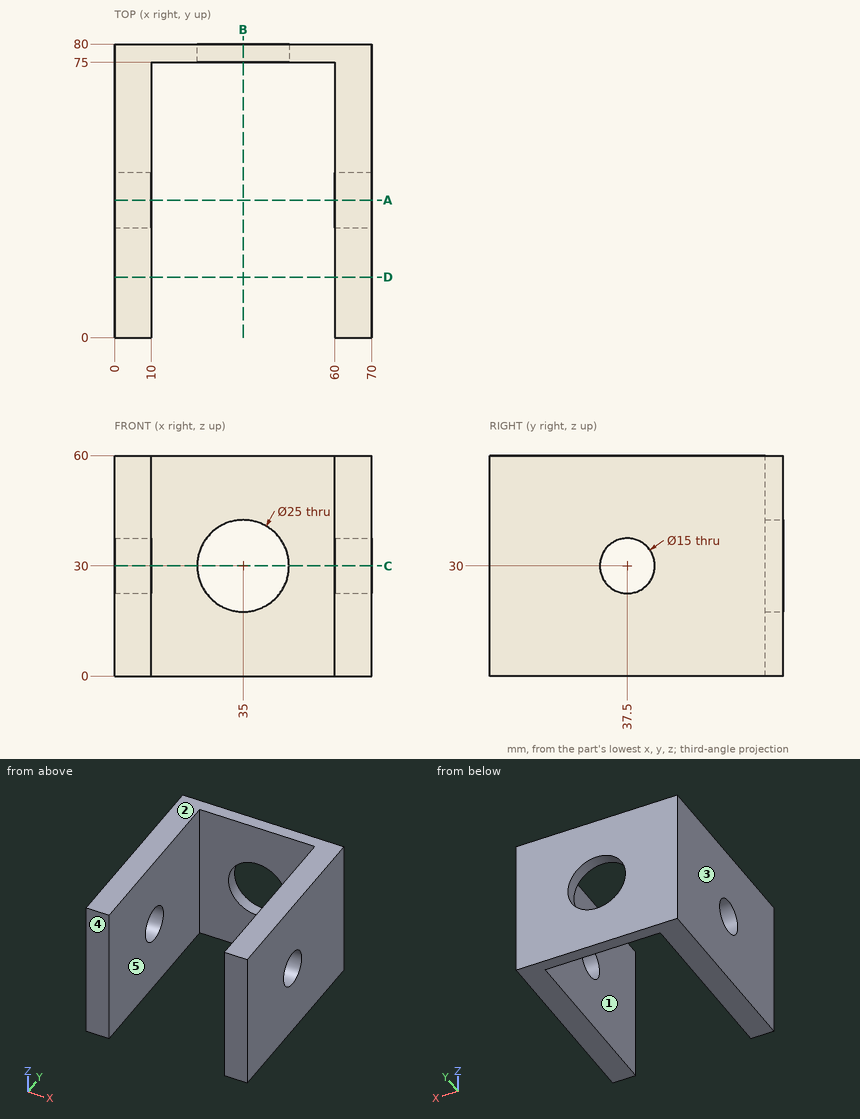
Source: three-view drawing plus pictorial views. Frame: mm from the lowest corner of the part. A direction names the side the tool comes from. Give positions to 0.01 mm unless a question says otherwise; leave off trailing zeros. Order: outer loops, then holes, each group sorted by start corner. A loop starts at its lowest first (then second) coordinate and runs counter-clockwise, first axis right, second up.
1. Mould query, pull axis X, two halves, no side actions, for the marked faces 3, 4 and 5. Classes: released by +X, released by -X, zero draft, split by the parting line, or undercut.
Derived:
face 3: released by -X
face 4: zero draft
face 5: undercut
2. Section D-D on y = 16.5. Return the cut outline in (x, z), and give its area (3 significant figures).
Derived:
outline: (0, 0) - (10, 0) - (10, 60) - (0, 60) - close; (60, 0) - (70, 0) - (70, 60) - (60, 60) - close
area: 1,200 mm2
3. Material intervals for L1, parallel to X at y = 22.5, z = 32; L2, parallel to Z at x = 35, y = 76.2; L3, parallel to Z at x = 64.75, y = 37.5, sorted ascending.
Derived:
L1: x = 0 to 10, 60 to 70
L2: z = 0 to 17.5, 42.5 to 60
L3: z = 0 to 22.5, 37.5 to 60
4. Pin query (flat end, axial travel): pin 1 (1 mm diameter, centred on x = 62, y = 71, fed in from -Z). Return the tip coordinate at first contact, or that it passes through.
Derived:
pin 1: stops at z = 0
5. Reachability of the marked faces 1 and 2 from +Z, -Z, +X, -X, +Y, -Y: full face, straight path, thin tool, end or side. Return the list, or none.
Derived:
face 1: +Z, -Z, -Y
face 2: +Z, +X, -X, +Y, -Y
6. Section C-C on z = 30. Return the cut outline in (x, y).
Derived:
outline: (0, 0) - (10, 0) - (10, 30) - (0, 30) - close; (0, 45) - (10, 45) - (10, 75) - (22.5, 75) - (22.5, 80) - (0, 80) - close; (47.5, 75) - (60, 75) - (60, 45) - (70, 45) - (70, 80) - (47.5, 80) - close; (60, 0) - (70, 0) - (70, 30) - (60, 30) - close
7. Section B-B on x = 35. Return the cut outline in (y, z).
Derived:
outline: (75, 0) - (80, 0) - (80, 17.5) - (75, 17.5) - close; (75, 42.5) - (80, 42.5) - (80, 60) - (75, 60) - close
8. Section A-A on y = 37.5. Return the cut outline in (x, z), and give its area (3 significant figures).
Derived:
outline: (0, 0) - (10, 0) - (10, 22.5) - (0, 22.5) - close; (0, 37.5) - (10, 37.5) - (10, 60) - (0, 60) - close; (60, 0) - (70, 0) - (70, 22.5) - (60, 22.5) - close; (60, 37.5) - (70, 37.5) - (70, 60) - (60, 60) - close
area: 900 mm2
